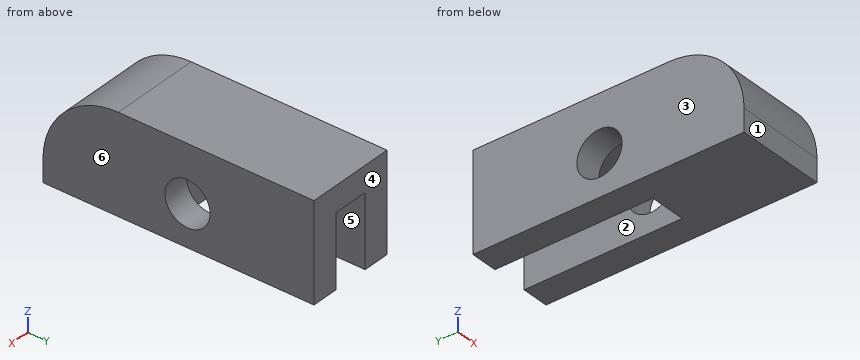
```python
from build123d import *

# Parameters (mm, degrees)
SKETCH2_W           = 16.51
SKETCH2_H           = 45.72
BOSS_EXTRUDE1_DEPTH = 7.62
FILLET1_R           = 12.7
SKETCH3_W           = 6.096
SKETCH3_H           = 26.67
CUT_EXTRUDE1_DEPTH  = 12.192
SKETCH4_R           = 3.81
CUT_EXTRUDE2_DEPTH  = 29.687666775


with BuildPart() as part:
    # Sketch2 → Boss-Extrude1 (new, symmetric)
    with BuildSketch(Plane(origin=(0, 0, 0), x_dir=(0, 0, -1), z_dir=(1, 0, 0))):
        Rectangle(SKETCH2_W, SKETCH2_H)
    extrude(amount=BOSS_EXTRUDE1_DEPTH, both=True)

    # Fillet1
    fillet1_edges = [part.edges().sort_by_distance(p)[0] for p in [
        (0, -22.86, 8.255),
    ]]
    fillet(fillet1_edges, radius=FILLET1_R)

    # Sketch3 → Cut-Extrude1 (cut)
    with BuildSketch(Plane(origin=(0, 0, -8.255), x_dir=(-1, 0, 0), z_dir=(0, 0, -1))):
        with Locations((0, 9.525)):
            Rectangle(SKETCH3_W, SKETCH3_H)
    extrude(amount=-CUT_EXTRUDE1_DEPTH, mode=Mode.SUBTRACT)

    # Sketch4 → Cut-Extrude2 (cut, through all)
    with BuildSketch(Plane(origin=(7.62, 0, 0), x_dir=(0, 0, -1), z_dir=(1, 0, 0))):
        with Locations((1.27, 1.524)):
            Circle(SKETCH4_R)
    extrude(amount=-CUT_EXTRUDE2_DEPTH, mode=Mode.SUBTRACT)


solid = part.part
```
Geometry: final body of the model. Coordinates: model frame, mm. Face numbers are marked on the shaded views. A direction names the side the tool comes from. Coordinates: 2 decimals unless noted, no trailing zeros. Order: outer loops, then holes, each group sorted by start corner. A loop starts at its lowest first (then second) coordinate and runs counter-clockwise, first axis right, second up. Notation, with made-up numbers: (86.5, 54) -> (109.5, 54) arc R22 cw to (109.5, 85) -> close; hole circle Ø1 at (-39.75, 81). An arc over 180 degrees is marked (long way). Answer in a Markdown table with one row per item.
Item 1: Section B-B on x = 2.5. Output: boundary loops of the cut face in (y, z) (3 decimals).
Return value:
| item | result |
|---|---|
| outline | (-22.86, -8.255) -> (-3.81, -8.255) -> (-3.81, 3.937) -> (22.86, 3.937) -> (22.86, 8.255) -> (-10.16, 8.255) arc R12.7 ccw to (-22.86, -4.445) -> close |
Item 2: Draft query along X for the marked faces 3, 4, 5 and 6. Return one class per face: released by +X, released by -X, zero draft, split by the parting line, or undercut.
Return value:
| item | result |
|---|---|
| face 3 | released by -X |
| face 4 | zero draft |
| face 5 | undercut |
| face 6 | released by +X |
Item 3: Ray query, L1, parallel to X at y = 11, z = 1; L2, parallel to Y at x = 5.05, z = -1.27; L3, parallel to Z at x = 6.25, y = -2 (3 decimals). Return the intervals inside material, ascending.
Return value:
| item | result |
|---|---|
| L1 | x = -7.62 to -3.05, 3.05 to 7.62 |
| L2 | y = -22.46 to -2.29, 5.33 to 22.86 |
| L3 | z = -8.255 to -2.718, 0.178 to 8.255 |
Item 4: Contact query for flat-ended pins moving along their axis: P1, Ø6, axis at y = 1.524, z = -1.27, coming from the +X side; P2, Ø5, axis at x = 4.5, z = 5.5, coming from the -Y side; P3, Ø1.8, axis at x = 1, z = -3.5, coming from the +Y side; P4, Ø3, axis at x = 1, y = 6, coming from the -Z side. Output: stop coordinate, or through.
Return value:
| item | result |
|---|---|
| P1 | passes through |
| P2 | stops at y = -20.45 |
| P3 | stops at y = -3.81 |
| P4 | stops at z = 3.94 |
Item 5: Access query for the marked faces 1 and 2. Directions: +Z, -Z, +X, -X, +Y, -Y. A direction counts if a zero-diameter tool reaches every point of the face in a straight line with its end or side. Return the directions, or none.
Return value:
| item | result |
|---|---|
| face 1 | +Z, -Z, +X, -X, -Y |
| face 2 | -Z, +Y |
Item 6: Section C-C on y = -0.5. Output: boundary loops of the cut face in (x, z) (3 decimals).
Return value:
| item | result |
|---|---|
| outline | (-7.62, -8.255) -> (-3.048, -8.255) -> (-3.048, -4.498) -> (-7.62, -4.498) -> close; (-7.62, 1.958) -> (-3.048, 1.958) -> (-3.048, 3.937) -> (3.048, 3.937) -> (3.048, 1.958) -> (7.62, 1.958) -> (7.62, 8.255) -> (-7.62, 8.255) -> close; (3.048, -8.255) -> (7.62, -8.255) -> (7.62, -4.498) -> (3.048, -4.498) -> close |
Item 7: Section A-A on z = -1.27. Output: boundary loops of the cut face in (x, y), plus the area to 3 significant figures.
Return value:
| item | result |
|---|---|
| outline | (-7.62, -22.46) -> (7.62, -22.46) -> (7.62, -2.29) -> (3.05, -2.29) -> (3.05, -3.81) -> (-3.05, -3.81) -> (-3.05, -2.29) -> (-7.62, -2.29) -> close; (-7.62, 5.33) -> (-3.05, 5.33) -> (-3.05, 22.86) -> (-7.62, 22.86) -> close; (3.05, 5.33) -> (7.62, 5.33) -> (7.62, 22.86) -> (3.05, 22.86) -> close |
| area | 458 mm² |
Item 8: Section D-D on y = 13.5. Output: boundary loops of the cut face in (x, z) (3 decimals), plus the area to 3 significant figures.
Return value:
| item | result |
|---|---|
| outline | (-7.62, -8.255) -> (-3.048, -8.255) -> (-3.048, 3.937) -> (3.048, 3.937) -> (3.048, -8.255) -> (7.62, -8.255) -> (7.62, 8.255) -> (-7.62, 8.255) -> close |
| area | 177 mm² |
